The drawing under review shows one solid part. Ordinate dimensions are in mm from its lowest x, y, z. Coordinates: 2 decimals unless noted, no trailing zeros. Write each loop counter-clockwise with the first axis right and the second up, starting at its lowest first coordinate (ties: lowest second). Pieces come first, ordered by that corner, then holes.
Q1. For probe 1 along X at (y, z) = (21.75, 19.5); probe 2 along Z at (x, y) = (6, 16.5); probe 3 along Z at (x, y) = (2.25, 24.25), list the stretches that pass through material, from the lowest coordinate up.
Q2. Take a section at C-C (z = 24.5). Give the boundary of the cut face in (x, y).
Q3. Take a section at B-B (x = 7). Give the boundary of the cut face in (y, z).
Q4. Take a section at A-A (y = 25.25). Give the boundary of the cut face in (x, z).
Q5. Insertion check: pin 1 (10 mm diameter, centred on x = 9, y = 10.5, fed in from +Z); pin 2 (1.5 mm diameter, centred on x = 11.5, y = 11, fed in from -Z); pin 3 (6 mm diameter, centred on x = 5, y = 17.5, fed in from -Z). Each pin has a flat end and moves straight along its axis. Give the tip position at first contact, or say it passes through.
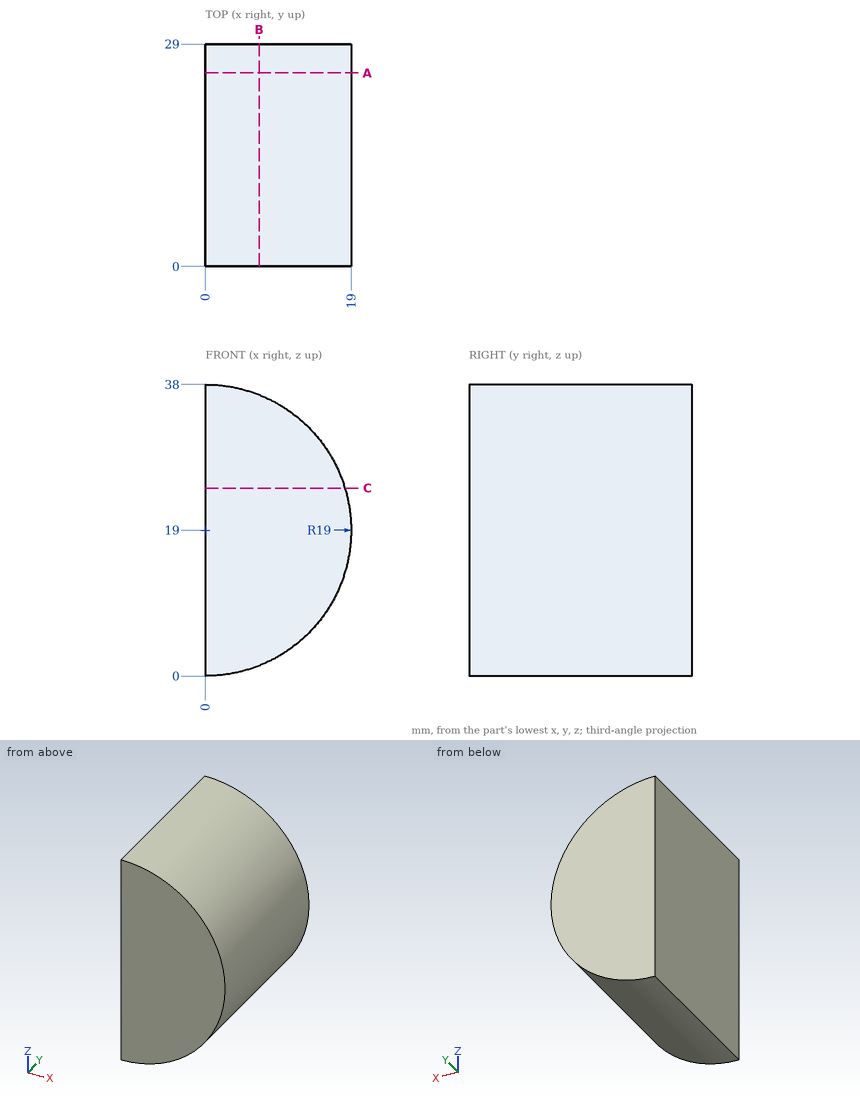
Response:
1. probe 1: x = 0 to 18.99
1. probe 2: z = 0.97 to 37.03
1. probe 3: z = 0.13 to 37.87
2. outline: (0, 0) - (18.19, 0) - (18.19, 29) - (0, 29) - close
3. outline: (0, 1.34) - (29, 1.34) - (29, 36.66) - (0, 36.66) - close
4. outline: (0, 0) arc R19 ccw to (0, 38) - close
5. pin 1: stops at z = 37.57
5. pin 2: stops at z = 3.33
5. pin 3: stops at z = 0.11
